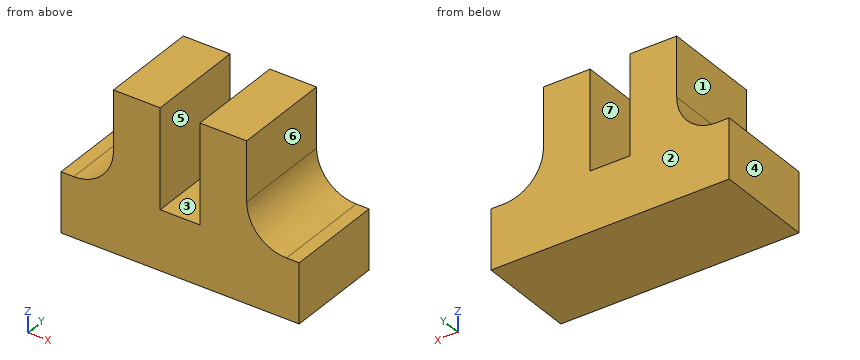
from build123d import *

# Parameters (mm, degrees)
F1_DEPTH = 15.875


with BuildPart() as f1:
    # F0 (on Front) → F1 (new body)
    with BuildSketch(Plane.XZ):
        with BuildLine():
            Line((-17.006651, 4.7625), (-19.05, 4.7625))
            Line((-19.05, 4.7625), (-19.05, -4.7625))
            Line((-19.05, -4.7625), (19.05, -4.7625))
            Line((19.05, -4.7625), (19.05, 4.7625))
            Line((19.05, 4.7625), (17.006651, 4.7625))
            ThreePointArc((17.006651, 4.7625), (12.516523, 6.622372), (10.656651, 11.1125))
            Line((10.656651, 11.1125), (10.656651, 20.6375))
            Line((10.656651, 20.6375), (3.175, 20.6375))
            Line((3.175, 20.6375), (3.175, 4.7625))
            Line((3.175, 4.7625), (-3.175, 4.7625))
            Line((-3.175, 4.7625), (-3.175, 20.6375))
            Line((-3.175, 20.6375), (-10.656651, 20.6375))
            Line((-10.656651, 20.6375), (-10.656651, 11.1125))
            ThreePointArc((-10.656651, 11.1125), (-12.516523, 6.622372), (-17.006651, 4.7625))
        make_face()
    extrude(amount=F1_DEPTH)


solid = f1.part
Check sheet for the modelled part. Datum: model origin and axes. Units: mm. Face numbers are marked on the shaded views. A direction names the side the tool comes from. Give positions to 0.01 mm unless a question says otherwise; leave off trailing zeros. Loops run counter-clockwise (first coordinate to the right, second up) from the corner with the lowest first, then second, coordinate; pieces in that order, holes last. Notation, with made-up numbers: M 36,79.25 L 59,79.25 A19 ccw 59,87.25 Z; hole C 78.5,78.5 d3. An arc over 180 degrees is marked long. Use a Markdown table: item, result. Add a question column.
Q1. Sectioned sample at D-D, the plane x = 14. Record the cut outline in (y, z) (1 decimal).
Q2. Tool access check on the marked faces 1, 2 and 3. Record the directions out of +Z, -Z, +X, -X, +Y, -Y that give a thin tool (end or side, any length) a straight path to the whole face; none if there is none.
Q3. Mould release check, pull along X, two halves, no side actions. Record for the marked faces 4, 5, 6 and 7: pulls with the +X half, pulls with the -X half, needs draft (parallel to the pull), parting line crosses it, or undercut.
Q4. Sectioned sample at A-A, the plane z = 14.5. Record the cut outline in (x, y) (3 decimals), then the cut area to 3 significant figures.
Q5. Scan lines: line 1 along X through (y, z) = (-7.75, 19.75) (3 decimals); line 2 along Z through (x, y) = (-1.5, -14); line 3 along X through (y, z) = (-12.5, 8.5) (3 decimals). Record each from-to range of solid material in increasing order. Write a range as [from, to].
Q6. Go/stop test with flat-tipped pins: pin 1 (7.5 mm diameter, centred on y = -9, z = 16, fed in from -X); pin 2 (1.6 mm diameter, centred on x = -18.5, y = -5, fed in from +Z); pin 3 (8 mm diameter, centred on y = -4, z = 14, fed in from +X). Record where each tip stops, or that it passes through.
Q7. Sectioned sample at C-C, the plane x = 0.5. Record the cut outline in (y, z) (1 decimal), then the cut area to 3 significant figures.
Verdict:
| question | item | result |
|---|---|---|
| 1 | outline | M -15.9,-4.8 L 0,-4.8 L 0,5.5 L -15.9,5.5 Z |
| 2 | face 1 | +Z, -X, +Y, -Y |
| 2 | face 2 | +Z, -Z, +X, -X, +Y |
| 2 | face 3 | +Z, +Y, -Y |
| 3 | face 4 | pulls with the -X half |
| 3 | face 5 | undercut |
| 3 | face 6 | pulls with the +X half |
| 3 | face 7 | undercut |
| 4 | outline | M -10.657,-15.875 L -3.175,-15.875 L -3.175,0 L -10.657,0 Z; M 3.175,-15.875 L 10.657,-15.875 L 10.657,0 L 3.175,0 Z |
| 4 | area | 238 mm^2 |
| 5 | line 1 | [-10.657, -3.175], [3.175, 10.657] |
| 5 | line 2 | [-4.76, 4.76] |
| 5 | line 3 | [-11.219, -3.175], [3.175, 11.219] |
| 6 | pin 1 | x = -10.66 |
| 6 | pin 2 | z = 4.76 |
| 6 | pin 3 | x = 10.75 |
| 7 | outline | M -15.9,-4.8 L 0,-4.8 L 0,4.8 L -15.9,4.8 Z |
| 7 | area | 151 mm^2 |
